Verification items for this drawing (mm, ordinates from the low corner). A direction names the side the tool comes from. Coordinates: 2 decimals unless noted, no trailing zeros. Order: outer loops, then holes, each group sorted by start corner. A loop starts at its lowest first (then second) coordinate and runs counter-clockwise, first axis right, second up. Notation, with made-up numbers: (67.5, -29) -> (123.5, -29) arc R11 ccw to (123.5, -10) -> close; hole circle Ø8 at (-33, 39). An arc over 180 degrees is marked (long way). Write item = value, one per line. Start each with the question number.
1. Set-up check for the marked faces 1 and 2: record each of +Z, -Z, +X, -X, +Y, -Y from which the full face is reachable in a straight line by a thin tool's end or side.
2. Cross-section at A-A on z = 3.15. Give the number of separate pieces and of enclosed holes in the cut face, plus the area to 3 significant figures.
3. Cross-section at D-D on z = 1.75. Record the cut outline in (x, y), plus the area to 3 significant figures.
4. Go/stop test with flat-tipped pins: P1, Ø2, axis at x = 21.5, y = 11, coming from the +Z side; P2, Ø0.8, axis at x = 7, z = 2, coming from the +Y side. Record where each tip stops, or that it passes through.
5. Thickness scan on line 1 along Y through (x, z) = (20.5, 2.7); line 2 along Z through (x, y) = (10.5, 16.25); line 3 along Z through (x, y) = (9.75, 1.75). Record the ranges inside material, lowest first. Write a range as from..to.
6. Cross-section at C-C on x = 13. Record the cut outline in (y, z), plus the area to 3 significant figures.
7. Cross-section at B-B on y = 2.25. Record the cut outline in (x, z), plus the area to 3 significant figures.
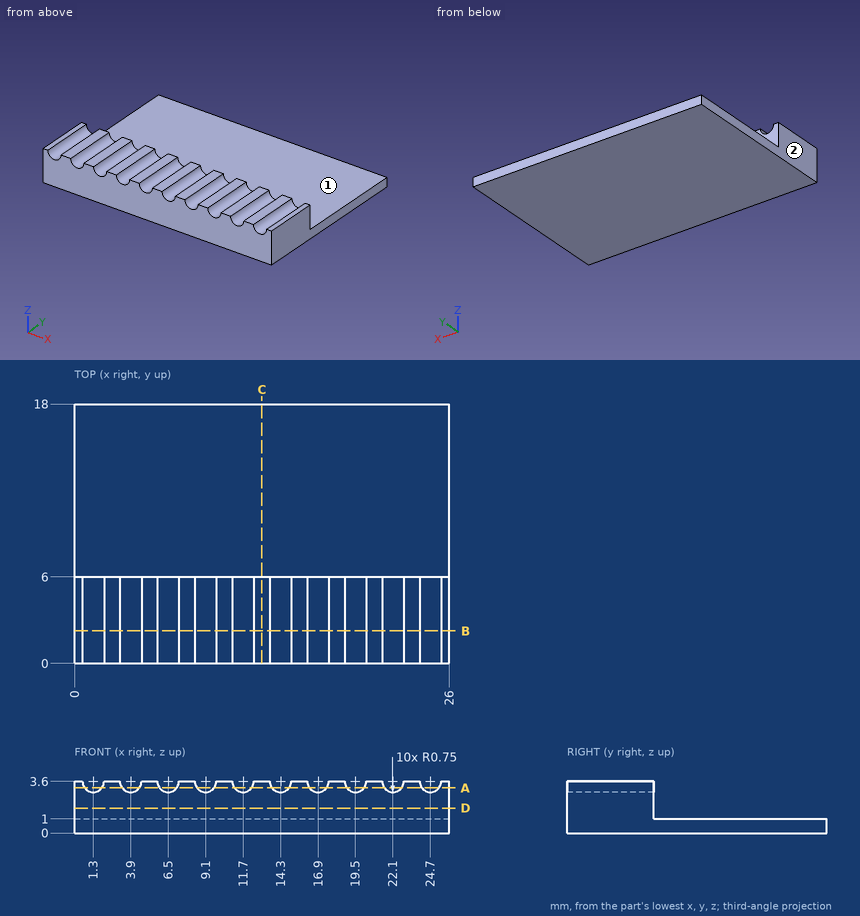
Worked out:
q1.face_1 = +Z, +X, -X, +Y
q1.face_2 = +Z, -Z, -X, +Y, -Y
q2.separate_pieces = 11
q2.enclosed_holes = 0
q2.area = 84.0 mm²
q3.outline = (0, 0) -> (26, 0) -> (26, 6) -> (0, 6) -> close
q3.area = 156 mm²
q4.P1 = 1
q4.P2 = 6
q5.line_1 = 0..6
q5.line_2 = 0..1
q5.line_3 = 0..3.23
q6.outline = (0, 0) -> (18, 0) -> (18, 1) -> (6, 1) -> (6, 3.6) -> (0, 3.6) -> close
q6.area = 33.6 mm²
q7.outline = (0, 0) -> (26, 0) -> (26, 3.6) -> (25.45, 3.6) arc R0.75 cw to (23.95, 3.6) -> (22.85, 3.6) arc R0.75 cw to (21.35, 3.6) -> (20.25, 3.6) arc R0.75 cw to (18.75, 3.6) -> (17.65, 3.6) arc R0.75 cw to (16.15, 3.6) -> (15.05, 3.6) arc R0.75 cw to (13.55, 3.6) -> (12.45, 3.6) arc R0.75 cw to (10.95, 3.6) -> (9.85, 3.6) arc R0.75 cw to (8.35, 3.6) -> (7.25, 3.6) arc R0.75 cw to (5.75, 3.6) -> (4.65, 3.6) arc R0.75 cw to (3.15, 3.6) -> (2.05, 3.6) arc R0.75 cw to (0.55, 3.6) -> (0, 3.6) -> close
q7.area = 84.8 mm²
